For this review, take the finished solid that the model builds, in its own axes (mm). A direction names the side the tool comes from. Give positions to 0.01 mm unless a question says otherwise; leave off trailing zeros. Loops run counter-clockwise (first coordinate to the right, second up) from the corner with the lowest first, then second, coordinate; pieces in that order, holes last. Notation, with made-up numbers: (67, 8.25) -> (92, 8.25) arc R20 cw to (92, 35.25) -> close; hole circle Ø9 at (39, 37.25). An arc over 180 degrees is marked (long way). Answer as CSV lines item,"result". Start each with the question number.
Item 1: Add section B-B on z = -7.75. State the section outline as (x, y) points.
Item 2: Machinability: for faces 1 (the face through (-1.2, 1, 8)), 2 (the face through (-0.1, 3.2, -2.8)), which of the approach directions +Z, -Z, +X, -X, +Y, -Y give a long, thin tool a straight path to every point of the face, cutting with its end or side? Answer none if there is none.
Item 3: Clearance check with flat-ended pins moving along their axes: P1, Ø1, axis at x = -10, y = 1.5, coming from the -Z side; P2, Ø3, axis at x = 7, y = 2, coming from the -Z side; P3, Ø1.6, axis at x = -7, y = 0.5, coming from the -Z side. State where each tip first meets the part, or that it passes through.
Item 4: For L1, parallel to Z at x = -0.5, y = 0.65; L2, parallel to Y at x = 1, z = -3.5; L3, parallel to X at y = 0.5, z = -10, list the stretches that pass through material, from the lowest coordinate up. Write a range as from..to.
Item 5: Add section C-C on x = 8. State the section outline as (y, z) points.
Item 6: The part is to be moulded in two halves that separate along Z. For faces 3 (the face through (-8, 3, 3.202)), 4 (the face through (0, 0, 0)), say which applies: +Z half, -Z half, draft (parallel to the pull), parting line (faces both ways), or undercut.
Item 7: Add section A-A on x = 0. State the section outline as (y, z) points, plus the area to 3 significant figures.
Item 8: Add section D-D on z = 4. State the section outline as (x, y) points.
```python
from build123d import *

# Parameters (mm, degrees)
CUT_EXTRUDE1_DEPTH = 21.420577857
CUT_EXTRUDE2_DEPTH = 3.5


with BuildPart() as part:
    # Sketch1 → Revolve1 (revolve)
    with BuildSketch(Plane.XY, mode=Mode.PRIVATE) as revolve1_sk:
        with BuildLine():
            Line((0, 0), (-14, 0))
            Line((-14, 0), (-14, 1))
            ThreePointArc((-14, 1), (-7.280109889, 3.980384612), (0, 5))
            Line((0, 5), (0, 0))
        make_face()
    revolve(revolve1_sk.sketch.rotate(Axis((0, 0, 0), (0, 1, 0)), 180), axis=Axis((0, 0, 0), (0, 1, 0)))

    # Sketch2 → Cut-Extrude1 (cut, through all)
    with BuildSketch(Plane(origin=(0, 5, 0), x_dir=(1, 0, 0), z_dir=(0, 1, 0))):
        with BuildLine():
            Line((1.2, 10), (1.2, 6))
            ThreePointArc((1.2, 6), (0, 4.8), (-1.2, 6))
            Line((-1.2, 6), (-1.2, 10))
            ThreePointArc((-1.2, 10), (0, 11.2), (1.2, 10))
        make_face()
        with BuildLine():
            Line((10, -1.2), (6, -1.2))
            ThreePointArc((6, -1.2), (4.8, 0), (6, 1.2))
            Line((6, 1.2), (10, 1.2))
            ThreePointArc((10, 1.2), (11.2, 0), (10, -1.2))
        make_face()
        with BuildLine():
            Line((-1.2, -10), (-1.2, -6))
            ThreePointArc((-1.2, -6), (0, -4.8), (1.2, -6))
            Line((1.2, -6), (1.2, -10))
            ThreePointArc((1.2, -10), (0, -11.2), (-1.2, -10))
        make_face()
        with BuildLine():
            Line((-10, 1.2), (-6, 1.2))
            ThreePointArc((-6, 1.2), (-4.8, 0), (-6, -1.2))
            Line((-6, -1.2), (-10, -1.2))
            ThreePointArc((-10, -1.2), (-11.2, 0), (-10, 1.2))
        make_face()
    extrude(amount=-CUT_EXTRUDE1_DEPTH, mode=Mode.SUBTRACT)

    # Sketch3 → Cut-Extrude2 (cut)
    with BuildSketch(Plane(origin=(0, 5, 0), x_dir=(1, 0, 0), z_dir=(0, 1, 0))):
        with BuildLine():
            Line((10.001792972, 3.197433741), (6.001792972, 3.197433741))
            ThreePointArc((6.001792972, 3.197433741), (2.801792972, -0.002566259), (6.001792972, -3.202566259))
            Line((6.001792972, -3.202566259), (10.001792972, -3.202566259))
            ThreePointArc((10.001792972, -3.202566259), (13.201792972, -0.002566259), (10.001792972, 3.197433741))
        make_face()
        with BuildLine():
            Line((3.2, 6), (3.2, 10))
            ThreePointArc((3.2, 10), (0, 13.2), (-3.2, 10))
            Line((-3.2, 10), (-3.2, 6))
            ThreePointArc((-3.2, 6), (0, 2.8), (3.2, 6))
        make_face()
        with BuildLine():
            Line((3.199226713, -10.004359231), (3.199226713, -6.004359231))
            ThreePointArc((3.199226713, -6.004359231), (-0.000773287, -2.804359231), (-3.200773287, -6.004359231))
            Line((-3.200773287, -6.004359231), (-3.200773287, -10.004359231))
            ThreePointArc((-3.200773287, -10.004359231), (-0.000773287, -13.204359231), (3.199226713, -10.004359231))
        make_face()
        with BuildLine():
            Line((-10.002566259, -3.201792972), (-6.002566259, -3.201792972))
            ThreePointArc((-6.002566259, -3.201792972), (-2.802566259, -0.001792972), (-6.002566259, 3.198207028))
            Line((-6.002566259, 3.198207028), (-10.002566259, 3.198207028))
            ThreePointArc((-10.002566259, 3.198207028), (-13.202566259, -0.001792972), (-10.002566259, -3.201792972))
        make_face()
    extrude(amount=-CUT_EXTRUDE2_DEPTH, mode=Mode.SUBTRACT)


solid = part.part
```
Computed values:
1,outline,"(-11.66, 0) -> (-1.2, 0) -> (-1.2, 1.5) -> (-3.2, 1.5) -> (-3.2, 3.64) arc R25.34 ccw to (-11.66, 1) -> close; (1.2, 0) -> (11.66, 0) -> (11.66, 1) arc R25.34 ccw to (3.2, 3.64) -> (3.2, 1.5) -> (1.2, 1.5) -> close"
2,face 1,"+Y, -Y"
2,face 2,"+Y"
3,P1,"z = -9.9"
3,P2,"z = -12.7"
3,P3,"z = -12.55"
4,L1,"-13.99..-11.09, -4.91..4.91, 11.09..13.99"
4,L2,"0..1.5"
4,L3,"-9.8..-1.2, 1.2..9.8"
5,outline,"(0, -11.49) -> (1, -11.49) arc R25.26 ccw to (3.56, -3.2) -> (1.5, -3.2) -> (1.5, -1.2) -> (0, -1.2) -> close; (0, 1.2) -> (1.5, 1.2) -> (1.5, 3.2) -> (3.56, 3.2) arc R25.26 ccw to (1, 11.49) -> (0, 11.49) -> close"
6,face 3,"undercut"
6,face 4,"draft"
7,outline,"(0, -14) -> (1, -14) arc R26.5 ccw to (1.5, -13.16) -> (1.5, -11.2) -> (0, -11.2) -> close; (0, -4.8) -> (1.5, -4.8) -> (1.5, -2.8) -> (4.85, -2.8) arc R26.5 ccw to (4.85, 2.8) -> (1.5, 2.8) -> (1.5, 4.8) -> (0, 4.8) -> close; (0, 11.2) -> (1.5, 11.2) -> (1.5, 13.16) arc R26.5 ccw to (1, 14) -> (0, 14) -> close"
7,area,"41.7 mm²"
8,outline,"(-13.42, 0) -> (13.42, 0) -> (13.42, 1) arc R26.2 ccw to (2.49, 4.58) -> (2.49, 1.5) -> (-2.5, 1.5) -> (-2.5, 4.58) arc R26.2 ccw to (-13.42, 1) -> close"
